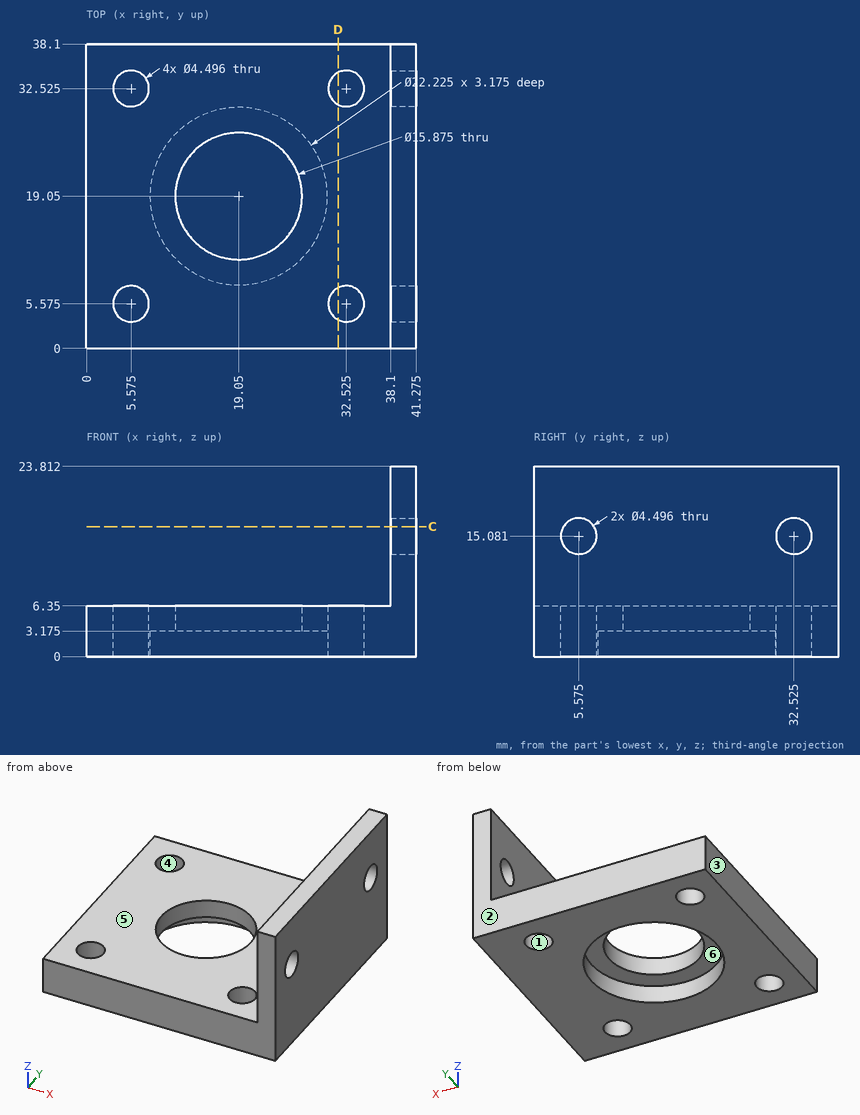
Source: three-view drawing plus pictorial views. Frame: mm from the lowest corner of the part. A direction names the side the tool comes from. Coordinates: 2 decimals unless noted, no trailing zeros. Loops run counter-clockwise (first coordinate to the right, second up) from the corner with the lowest first, then second, coordinate; pieces in that order, holes last. Notation, with made-up numbers: (-4, -5.75) - (48, -5.75) arc R13 cw to (48, 16.25) - close; hole circle Ø10 at (66.5, 44.25). An arc over 180 degrees is marked (long way). One line per item, written item: value. Start each with the question number.
1. Set-up query: the marked faces 4, 5 and 6. Return all of +Z, -Z, +X, -X, +Y, -Y with unobstructed straight access to the full face (end or side cutting, diameter ignored); none if empty.
2. Contact query for flat-ended pins moving along their axis: P1, Ø5, axis at y = 23.5, z = 18, coming from the -X side; P2, Ø4, axis at x = 5.58, y = 5.58, coming from the -Z side; P3, Ø2, axis at x = 6, y = 21.5, coming from the +Z side. Output: stop coordinate, or through.
3. Mould query, pull axis X, two halves, no side actions, for the marked faces 1, 2 and 3. Classes: pulls with the +X half, pulls with the -X half, needs draft (parallel to the pull), parting line crosses it, or undercut.
4. Ray query, L1, parallel to Y at x = 7, z = 6 (1 decimal); L2, parallel to Z at x = 7, y = 10.5; L3, parallel to X at y = 8, z = 14 (1 decimal). Return the intervals inside material, ascending.
5. Section D-D (x = 31.5). State how many separate pieces and enclosed holes the cut face has, and give its area (3 significant figures).
6. Section C-C (z = 16.25). Return the cut outline in (x, y) (1 decimal).
Verdict:
1. face 4: +Z, -Z
1. face 5: +Z, -X, +Y, -Y
1. face 6: -Z
2. P1: stops at x = 38.1
2. P2: passes through
2. P3: stops at z = 6.35
3. face 1: undercut
3. face 2: needs draft
3. face 3: pulls with the -X half
4. L1: y = 0 to 3.8, 7.3 to 30.8, 34.3 to 38.1
4. L2: z = 0 to 6.35
4. L3: x = 38.1 to 41.3
5. separate pieces: 3
5. enclosed holes: 0
5. area: 191 mm2
6. outline: (38.1, 0) - (41.3, 0) - (41.3, 3.7) - (38.1, 3.7) - close; (38.1, 7.5) - (41.3, 7.5) - (41.3, 30.6) - (38.1, 30.6) - close; (38.1, 34.4) - (41.3, 34.4) - (41.3, 38.1) - (38.1, 38.1) - close
